```python
from build123d import *

# Parameters (mm, degrees)
STOCK_LEFT_START                     = 6602.1458
STOCK_LEFT_CONSOLE_1_OUTLINE_R       = 2.286
STOCK_LEFT_CONSOLE_1_OUTLINE_R_2     = 44.45
STOCK_LEFT_CONSOLE_1_DEPTH           = 19.05
SKETCH1_R                            = 2.286
BOSS_EXTRUDE1_DEPTH                  = 19.05
F_5_64_0_07813_DIAMETER_HOLE1_D      = 1.984502
F_5_64_0_07813_DIAMETER_HOLE1_DEPTH  = 38.1
F_5_64_0_07813_DIAMETER_HOLE1_TIP    = 0.59620455
HOLE1_D                              = 1.98374
HOLE1_DEPTH                          = 19.05
HOLE1_CSINK_D                        = 10.16
HOLE1_CSINK_ANGLE                    = 82
HOLE1_TIP                            = 0.595975622
F_15_64_0_23438_DIAMETER_HOLE1_D     = 5.953252
F_15_64_0_23438_DIAMETER_HOLE1_DEPTH = 12.7
F_15_64_0_23438_DIAMETER_HOLE1_TIP   = 1.788537341
F_15_64_0_23438_DIAMETER_HOLE2_D     = 5.953252


# Read off the part's stored shape, not the designer's step: Stock-Left Console-1
with BuildPart() as part:
    # Stock-Left Console-1 outline → Stock-Left Console-1 (new body)
    with BuildSketch(Plane(origin=(0, 0, 0), x_dir=(1, 0, 0), z_dir=(0, 1, 0)).offset(STOCK_LEFT_START)):
        with BuildLine():
            Line((357.802906487, -3322.246193472), (427.81043067, -3322.246195127))
            add(Edge.make_bspline(
                [(427.81043067, -3322.246195127), (473.388143546, -3207.192047458), (498.434160064, -3084.558176537), (504.840097902, -2846.856520671), (500.419755279, -2759.632030412), (493.181235291, -2683.510000386)],
                knots=[-62.01580073, -62.01580073, -62.01580073, -62.01580073, -27.97842461, -27.97842461, -9.154068647, -9.154068647, -9.154068647, -9.154068647], degree=3))
            Line((493.181235291, -2683.510000386), (273.05, -2683.510000011))
            Line((273.05, -2683.510000011), (273.05, -2933.697739453))
            Line((273.05, -2933.697739453), (298.063657014, -2938.111010516))
            Line((298.063657014, -2938.111010516), (314.509168719, -2844.900694709))
            ThreePointArc((314.509168719, -2844.900694709), (329.148175534, -2829.611779383), (348.875396841, -2837.285643591))
            Line((348.875396841, -2837.285643591), (418.46673346, -2936.69442468))
            ThreePointArc((418.46673346, -2936.69442468), (430.437407433, -2963.905621235), (431.085143003, -2993.626433673))
            Line((431.085143003, -2993.626433673), (427.658008361, -3013.062680059))
            Line((427.658008361, -3013.062680059), (459.43413222, -3018.669083307))
            add(Edge.make_bspline(
                [(459.43413222, -3018.669083307), (456.223775647, -3054.466127933), (451.650547457, -3088.445708947), (445.737069512, -3121.041687467), (439.008868755, -3158.128540481), (430.553849402, -3193.432616991), (420.351653238, -3227.631207238)],
                knots=[34.96272562, 34.96272562, 34.96272562, 34.96272562, 43.828946319, 43.828946319, 43.828946319, 53.916700663, 53.916700663, 53.916700663, 53.916700663], degree=3))
            Line((420.351653238, -3227.631207238), (357.739033333, -3290.49625772))
            Line((357.739033333, -3290.49625772), (357.802906487, -3322.246193472))
        make_face()
        with Locations((373.658776627, -3312.721193497)):
            Circle(STOCK_LEFT_CONSOLE_1_OUTLINE_R, mode=Mode.SUBTRACT)
        with Locations((411.758776627, -3312.721193478)):
            Circle(STOCK_LEFT_CONSOLE_1_OUTLINE_R, mode=Mode.SUBTRACT)
        with Locations((463.209250621, -3010.106955909)):
            Circle(STOCK_LEFT_CONSOLE_1_OUTLINE_R, mode=Mode.SUBTRACT)
        with Locations((486.003084481, -3006.374869262)):
            Circle(STOCK_LEFT_CONSOLE_1_OUTLINE_R, mode=Mode.SUBTRACT)
        with Locations((287.824193289, -2929.856338812)):
            Circle(STOCK_LEFT_CONSOLE_1_OUTLINE_R, mode=Mode.SUBTRACT)
        with Locations((279.4, -2915.847898591)):
            Circle(STOCK_LEFT_CONSOLE_1_OUTLINE_R, mode=Mode.SUBTRACT)
        with Locations((292.1, -2727.960000043)):
            Circle(STOCK_LEFT_CONSOLE_1_OUTLINE_R, mode=Mode.SUBTRACT)
        with Locations((292.1, -2702.559999968)):
            Circle(STOCK_LEFT_CONSOLE_1_OUTLINE_R, mode=Mode.SUBTRACT)
        with Locations((317.5, -2702.559999968)):
            Circle(STOCK_LEFT_CONSOLE_1_OUTLINE_R, mode=Mode.SUBTRACT)
        with Locations((443.068858037, -2998.799793605)):
            Circle(STOCK_LEFT_CONSOLE_1_OUTLINE_R, mode=Mode.SUBTRACT)
        with Locations((392.883884122, -2772.410060986)):
            Circle(STOCK_LEFT_CONSOLE_1_OUTLINE_R_2, mode=Mode.SUBTRACT)
        with Locations((450.85, -2727.960000048)):
            Circle(STOCK_LEFT_CONSOLE_1_OUTLINE_R, mode=Mode.SUBTRACT)
        with Locations((450.85, -2702.560000048)):
            Circle(STOCK_LEFT_CONSOLE_1_OUTLINE_R, mode=Mode.SUBTRACT)
    extrude(amount=STOCK_LEFT_CONSOLE_1_DEPTH)

    # Sketch1 → Boss-Extrude1 (add)
    with BuildSketch(Plane(origin=(0, 6621.1958, 0), x_dir=(1, 0, 0), z_dir=(0, 1, 0))):
        with Locations((292.1, -2727.959998746)):
            Circle(SKETCH1_R)
        with Locations((292.1, -2702.559998672)):
            Circle(SKETCH1_R)
        with Locations((317.5, -2702.559998672)):
            Circle(SKETCH1_R)
        with Locations((450.85, -2702.559998751)):
            Circle(SKETCH1_R)
        with Locations((450.85, -2727.959998751)):
            Circle(SKETCH1_R)
    extrude(amount=-BOSS_EXTRUDE1_DEPTH)

    # 5/64 (0.07813) Diameter Hole1
    with Locations(Plane(origin=(0, 0, 2664.46), x_dir=(-1, 0, 0), z_dir=(0, 0, -1))):
        with Locations((-481.589248274, 6993.254992531), (-386.339248274, 6993.254992531), (-291.089248274, 6993.254992531), (-295.274999999, 6965.135938475), (-295.274999999, 6812.735938475), (-295.274999999, 6660.335938474), (-285.166362357, 6631.468843414), (-475.477307398, 6631.468752771), (-485.002307398, 6660.335938474), (-485.002307398, 6812.735938474), (-485.002307398, 6965.135938474), (-478.365617646, 6611.6708), (-287.865617646, 6611.6708), (-307.975, 6564.3379), (-307.975, 6488.1379), (-284.960913066, 6440.805), (-380.210913066, 6440.805), (-475.460913066, 6440.805), (-446.831312422, 6488.1379), (-446.831312422, 6564.3379), (-472.231312422, 6396.355), (-472.231312422, 6320.155), (-472.653156211, 6275.705000839), (-377.403156211, 6275.705000839), (-282.153156211, 6275.705000839), (-282.575, 6320.155), (-282.575, 6396.355), (-435.598646187, 6221.729999816), (-435.598646187, 6145.529999816), (-450.592518112, 6091.554999951), (-460.998646187, 6091.555478285), (-460.998646187, 6056.629999944), (-460.998646187, 5980.429999944), (-460.998646187, 5945.505000042), (-282.153156211, 5945.505000042), (-368.611823093, 5945.505000042)):
            Hole(F_5_64_0_07813_DIAMETER_HOLE1_D / 2, depth=F_5_64_0_07813_DIAMETER_HOLE1_DEPTH)
            with Locations((0, 0, -(F_5_64_0_07813_DIAMETER_HOLE1_DEPTH + F_5_64_0_07813_DIAMETER_HOLE1_TIP / 2))):  # 118° drill point
                Cone(0, F_5_64_0_07813_DIAMETER_HOLE1_D / 2, F_5_64_0_07813_DIAMETER_HOLE1_TIP, mode=Mode.SUBTRACT)

    # Hole1
    with Locations(Plane(origin=(0, 6621.1958, 0), x_dir=(1, 0, 0), z_dir=(0, 1, 0))):
        with Locations((307.975, -2724.785), (307.975, -2708.91), (446.831312422, -2724.785), (446.831312422, -2708.91)):
            CounterSinkHole(HOLE1_D / 2, HOLE1_CSINK_D / 2, depth=HOLE1_DEPTH, counter_sink_angle=HOLE1_CSINK_ANGLE)
            with Locations((0, 0, -(HOLE1_DEPTH + HOLE1_TIP / 2))):  # 118° drill point
                Cone(0, HOLE1_D / 2, HOLE1_TIP, mode=Mode.SUBTRACT)

    # 15/64 (0.23438) Diameter Hole1
    with Locations(Plane.ZY.offset(-273.05)):
        with Locations((2746.056935059, 6611.6708), (2871.150804655, 6611.6708)):
            Hole(F_15_64_0_23438_DIAMETER_HOLE1_D / 2, depth=F_15_64_0_23438_DIAMETER_HOLE1_DEPTH)
            with Locations((0, 0, -(F_15_64_0_23438_DIAMETER_HOLE1_DEPTH + F_15_64_0_23438_DIAMETER_HOLE1_TIP / 2))):  # 118° drill point
                Cone(0, F_15_64_0_23438_DIAMETER_HOLE1_D / 2, F_15_64_0_23438_DIAMETER_HOLE1_TIP, mode=Mode.SUBTRACT)

    # 15/64 (0.23438) Diameter Hole2 (through all)
    with Locations(Plane(origin=(0, 6621.1958, 0), x_dir=(1, 0, 0), z_dir=(0, 1, 0))):
        with Locations((439.860441392, -3210.015746304), (449.077665614, -3173.047479133)):
            Hole(F_15_64_0_23438_DIAMETER_HOLE2_D / 2)


solid = part.part
```
Could you check a few things on this model? Use its own coordinates, in mm. A direction names the side the tool comes from. Coordinates: 2 decimals unless noted, no trailing zeros. Put each result on its own line as item: value. Start each with the question number.
(1) For faces 4 (the face through (389.484, 6611.537, 3258.624)), 5 (the face through (392, 6612, 3322.246)), 6 (the face through (306.17, 6611.54, 2892.16)), which set-ups out of +Z, -Z, +X, -X, +Y, -Y let a thin tool reach every point of the face, with its end or its side?
(2) Thinking about a two-plate mould opening in X: for faces 1 (the face through (383.18, 6611.54, 2886.29)), 2 (the face through (413, 6602.146, 2856)), 3 (the face through (443.324, 6611.537, 3015.827)), which applies, pulls with the +X half, pulls with the -X half, needs draft (parallel to the pull), parting line crosses it, or undercut?
(3) Will these pins go through, and if not, where does the flat tip stop? P1, Ø1.8, axis at x = 287.87, y = 6611.67, coming from the -Z side; P2, Ø2.5, axis at x = 446.83, z = 2708.91, coming from the +Y side; P3, Ø4, axis at y = 6615.5, z = 3004, coming from the -X side.
(4) I need wall thicknesses on line 1 (Z direction, x = 409, y = 6607.5); line 2 (Z direction, x = 377.5, y = 6607.5); line 3 (X direction, y = 6605.5, z = 2794). Which ranges of each line are inside material? Lowest first, please. Write a range as from..to.
Solutions:
1. face 4: -X, +Y, -Y
1. face 5: +Z, +X, -X, +Y, -Y
1. face 6: +Z, +Y, -Y
2. face 1: undercut
2. face 2: needs draft
2. face 3: pulls with the -X half
3. P1: stops at z = 2702.61
3. P2: stops at y = 6616.79
3. P3: stops at x = 428.9
4. line 1: z = 2683.51..2730.98, 2813.84..2923.17, 3239.03..3322.25
4. line 2: z = 2683.51..2730.71, 2814.11..2878.17, 3270.66..3322.25
4. line 3: x = 273.05..354.03, 431.74..500.99
